from build123d import *

# Parameters (mm, degrees)
BOSS_EXTRUDE1_DEPTH = 3.0988
SKETCH3_R           = 1.0795
SKETCH3_R_2         = 11.6713
BOSS_EXTRUDE2_DEPTH = 3.0988
CUT_EXTRUDE1_DEPTH  = 122.505558808
FILLET1_R           = 5.08


with BuildPart() as part:
    # Sketch2 → Boss-Extrude1 (new body)
    with BuildSketch(Plane.XY):
        Polygon((-50.8, 1.5494), (-50.8, 7.8994), (50.8, 7.8994), (50.8, -7.8994), (-50.8, -7.8994), (-50.8, -1.5494), (0, -1.5494), (0, 1.5494), align=None)
    extrude(amount=BOSS_EXTRUDE1_DEPTH)

    # Sketch3 → Boss-Extrude2 (add)
    with BuildSketch(Plane.XY):
        with BuildLine():
            Line((50.8, -7.8994), (-50.8, -7.8994))
            Line((-50.8, -7.8994), (-50.8, -20.5994))
            Line((-50.8, -20.5994), (101.6, -20.5994))
            Line((101.6, -20.5994), (101.6, 33.2994))
            Line((101.6, 33.2994), (54.782161872, 63.523702231))
            ThreePointArc((54.782161872, 63.523702231), (46.597523005, 66.447615713), (37.96588061, 65.431577828))
            Line((37.96588061, 65.431577828), (-50.8, 33.2994))
            Line((-50.8, 33.2994), (-50.8, 7.8994))
            Line((-50.8, 7.8994), (50.8, 7.8994))
            Line((50.8, 7.8994), (50.8, -7.8994))
        make_face()
        with Locations((76.2, 0)):
            Circle(SKETCH3_R, mode=Mode.SUBTRACT)
        with Locations((44.45, 47.519048812)):
            Circle(SKETCH3_R_2, mode=Mode.SUBTRACT)
    extrude(amount=BOSS_EXTRUDE2_DEPTH)

    # Sketch4 → Cut-Extrude1 (cut, through all)
    with BuildSketch(Plane.XY.offset(3.0988)):
        with BuildLine():
            ThreePointArc((63.5, 47.519048812), (63.232160807, 44.33582161), (62.436174759, 41.242105484))
            Line((62.436174759, 41.242105484), (50.8, 7.8994))
            Line((50.8, 7.8994), (50.8, -20.5994))
            Line((50.8, -20.5994), (101.6, -20.5994))
            Line((101.6, -20.5994), (101.6, 33.2994))
            Line((101.6, 33.2994), (54.782161872, 63.523702231))
            ThreePointArc((54.782161872, 63.523702231), (61.179168892, 56.6315352), (63.5, 47.519048812))
        make_face()
    extrude(amount=-CUT_EXTRUDE1_DEPTH, mode=Mode.SUBTRACT)

    # Fillet1
    fillet1_edges = [part.edges().sort_by_distance(p)[0] for p in [
        (-50.8, 33.2994, 1.5494),
        (-50.8, -20.5994, 1.5494),
        (50.8, -20.5994, 1.5494),
        (50.8, 7.8994, 1.5494),
    ]]
    fillet(fillet1_edges, radius=FILLET1_R)


solid = part.part
The listing builds one solid part. Answer for the finished solid, in the listing's coordinates (mm). A direction names the side the tool comes from. Give positions to 0.01 mm unless a question says otherwise; leave off trailing zeros. Write each loop counter-clockwise with the first axis right and the second up, starting at its lowest first coordinate (ties: lowest second). Pieces come first, ordered by that corner, then holes.
1) Section B-B (z = 1.15) is taken. Write down the section's boundary in (x, y), and give its area (3 significant figures).
2) Given P1, Ø0.9, axis at x = -33, z = 2, coming from the +Y side; P2, Ø1, axis at y = 51, z = 2.5, coming from the +X side; P3, Ø0.9, axis at y = 0, z = 2, coming from the -X side, each flat-ended and moving along its own axis, determine where each tip first touches the part or whether it passes through.
3) Section A-A (x = 44.45) is taken. Write down the section's boundary in (y, z).
4) Find the intervals of material crossed by L1, parallel to Y at x = 44.45, z = 1.7; L2, parallel to Y at x = -11.5, z = 2.15; L3, parallel to X at y = 6.5, z = 1.75, in increasing order.
5) A tool of negligible diameter and unlimited length cuts with its end or side. For faces 5 (the face through (50.8, -4, 2)), 6 (the face through (0, 0, 2)), 7 (the face through (-1, -20.599, 2)), from which of +Z, -Z, +X, -X, +Y, -Y can it reach the whole face along a straight path? Write none if from no direction.
6) Section C-C (y = 58) is taken. Write down the section's boundary in (x, z).
7) For a pull along Y with two mould halves and no side action, classify faces 1 (the face through (-25, 1.549, 2)), 2 (the face through (-49.9, 32.62, 1.57)), 3 (the face through (56.839, 25.205, 1.571)), 4 (the face through (-50.8, 16, 2)) as pulls with the +Y half, pulls with the -Y half, needs draft (parallel to the pull), parting line crosses it, or undercut.
8) Section D-D (y = -9) is taken. Write down the section's boundary in (x, z).
Response:
1. outline: (-50.8, -15.52) arc R5.08 ccw to (-45.72, -20.6) - (45.72, -20.6) arc R5.08 ccw to (50.8, -15.52) - (50.8, 7.04) arc R5.08 cw to (51.08, 8.71) - (62.44, 41.24) arc R19.05 ccw to (37.97, 65.43) - (-47.45, 34.51) arc R5.08 ccw to (-50.8, 29.74) - (-50.8, 1.55) - (0, 1.55) - (0, -1.55) - (-50.8, -1.55) - close; hole circle Ø23.34 at (44.45, 47.52)
1. area: 7,160 mm2
2. P1: stops at y = 39.91
2. P2: stops at x = 63.27
2. P3: stops at x = 0
3. outline: (-20.6, 0) - (35.85, 0) - (35.85, 3.1) - (-20.6, 3.1) - close; (59.19, 0) - (66.57, 0) - (66.57, 3.1) - (59.19, 3.1) - close
4. L1: y = -20.6 to 35.85, 59.19 to 66.57
4. L2: y = -20.6 to -1.55, 1.55 to 47.53
4. L3: x = -50.8 to 50.8
5. face 5: +Z, -Z, +X, -Y
5. face 6: +Z, -Z, -X
5. face 7: +Z, -Z, +X, -X, -Y
6. outline: (17.44, 0) - (39.31, 0) - (39.31, 3.1) - (17.44, 3.1) - close; (49.59, 0) - (60.36, 0) - (60.36, 3.1) - (49.59, 3.1) - close
7. face 1: undercut
7. face 2: pulls with the +Y half
7. face 3: pulls with the -Y half
7. face 4: needs draft
8. outline: (-50.8, 0) - (50.8, 0) - (50.8, 3.1) - (-50.8, 3.1) - close
